Could you check a few things on this model? Use its own coordinates, in mm. Face numbers are marked on the shaded views. A direction names the side the tool comes from. Give positions to 0.01 mm unless a question says otherwise; leave off trailing zeros. Loops run counter-clockwise (first coordinate to the right, second up) from the corner with the lowest first, then second, coordinate; pieces in that order, holes last. Notation, with made-up numbers: M -37,63.5 L -27,63.5 A23 cw -27,87.5 Z; hole C -24.5,73.25 d4. An arc over 180 degrees is marked long. Use CSV: the item, a comma, the result in double quotes.
Autodesk Inventor part; units mm, degrees
ref_plane "Work Plane2" through (0, 7.92, 0) normal (0, 1, 0) x (1, 0, 0)
ref_plane "Work Plane3" through (0, 3.42, 0) normal (0, 1, 0) x (1, 0, 0)
ref_plane "YZ Plane" through (0, 0, 0) normal (1, 0, 0) x (0, 1, 0)
sketch "Sketch1" plane through (0, 0, 0) normal (0, 1, 0) x (-1, 0, 0)
  circle A0 centre (0, 0) radius 7
  dimension "d0" = 14
extrude "Extrusion1" add sketch "Sketch1" along normal blind 2.12
sketch "Sketch3" plane through (0, 2.12, 0) normal (0, 1, 0) x (1, 0, 0)
  circle A0 centre (0, 0) radius 4.5
  dimension "d4" = 9
extrude "Extrusion2" add sketch "Sketch3" along normal blind 1.3
ref_plane "Work Plane2" through (0, 7.92, 0) normal (0, 1, 0) x (1, 0, 0)
sketch "Sketch5" plane through (0, 7.92, 0) normal (0, 1, 0) x (1, 0, 0)
  circle A0 centre (0, 0) radius 7
  dimension "d8" = 14
loft "Loft1" add profiles "Sketch5" section 1 edges at (-4.5, 3.42, 0)
sketch "Sketch7" plane through (0, 7.92, 0) normal (0, 1, 0) x (1, 0, 0)
  circle A0 centre (0, 0) radius 7
extrude "Extrusion3" add sketch "Sketch7" along normal blind 1.6
sketch "Sketch8" plane through (0, 9.52, 0) normal (0, 1, 0) x (1, 0, 0)
  circle A0 centre (0, 0) radius 5.2
  dimension "d15" = 10.4
ref_plane "Work Plane3" through (0, 3.42, 0) normal (0, 1, 0) x (1, 0, 0)
sketch "Sketch10" plane through (0, 3.42, 0) normal (0, 1, 0) x (1, 0, 0)
  circle A0 centre (0, 0) radius 1.85
  dimension "d22" = 3.7
loft "Loft3" cut profiles "Sketch8", "Sketch10"
hole "Hole1" at (0, 0, 0) direction (0, 1, 0) diameter 3.7 end through all
equation "\"d34\" = Thickness"
equation "\"BendRadius\" = Thickness"
equation "\"BendReliefWidth\" = Thickness"
equation "\"BendReliefDepth\" = 0.5 * Thickness"
equation "\"CornerReliefSize\" = 4 * Thickness"
equation "\"MinimumRemnant\" = 2 * Thickness"
equation "\"TransitionRadius\" = BendRadius"
equation "\"JacobiRadiusSize\" = Thickness"
equation "\"GapSize\" = Thickness"
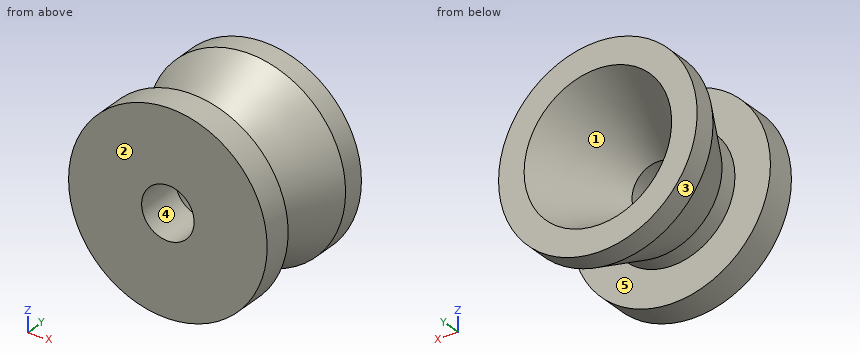
1. Please list where these lines run through material, in increasing order: line 1 (Z direction, x = 0, y = 2.35); line 2 (Z direction, x = 0, y = 1); line 3 (Y direction, x = 5.5, z = 2.5).
Outcome:
line 1,"-4.5 to -1.85, 1.85 to 4.5"
line 2,"-7 to -1.85, 1.85 to 7"
line 3,"0 to 2.12, 6.19 to 9.52"
2. I want a section at C-C, the plane y = 1. List the corners of the cut face in (x, z) for me.
Outcome:
outline,"C 0,0 d14; hole C 0,0 d3.7"
3. Which directions (+Z, -Z, +X, -X, +Y, -Y) give clear straight access to the entire face, cutting with the end or side of a thin tool? Please do the marked faces 4 and 5.
Outcome:
face 4,"+Y, -Y"
face 5,"none"
4. I want a section at B-B, the plane y = 2.75. List the corners of the cut face in (x, z) for me.
Outcome:
outline,"C 0,0 d9; hole C 0,0 d3.7"
5. I'm going to push flat-ended pins straight in: pin 1 Ø2 at (y, z) = (6.5, 5.5) entering from -X; pin 2 Ø1.5 at (x, z) = (0.5, 2.5) entering from +Y; pin 3 Ø1 at (x, y) = (3, 1.5) entering from -Z. Where does each tip first touch, or does it pass through?
Outcome:
pin 1,"x = -4.55"
pin 2,"y = 6.06"
pin 3,"z = -6.54"
6. I want a section at A-A, the plane x = 0. List the corners of the cut face in (y, z) for me.
Outcome:
outline,"M 0,-7 L 2.12,-7 L 2.12,-4.5 L 3.42,-4.5 L 7.92,-7 L 9.52,-7 L 9.52,-5.2 L 3.42,-1.85 L 0,-1.85 Z; M 0,1.85 L 3.42,1.85 L 9.52,5.2 L 9.52,7 L 7.92,7 L 3.42,4.5 L 2.12,4.5 L 2.12,7 L 0,7 Z"
7. If we mould it in two halves opening along Z, with no side actions, what happens to the marked faces 1, 2 and 3? For each: +Z half, -Z half, draft (parallel to the pull), parting line (faces both ways), or undercut.
Outcome:
face 1,"undercut"
face 2,"draft"
face 3,"parting line"
